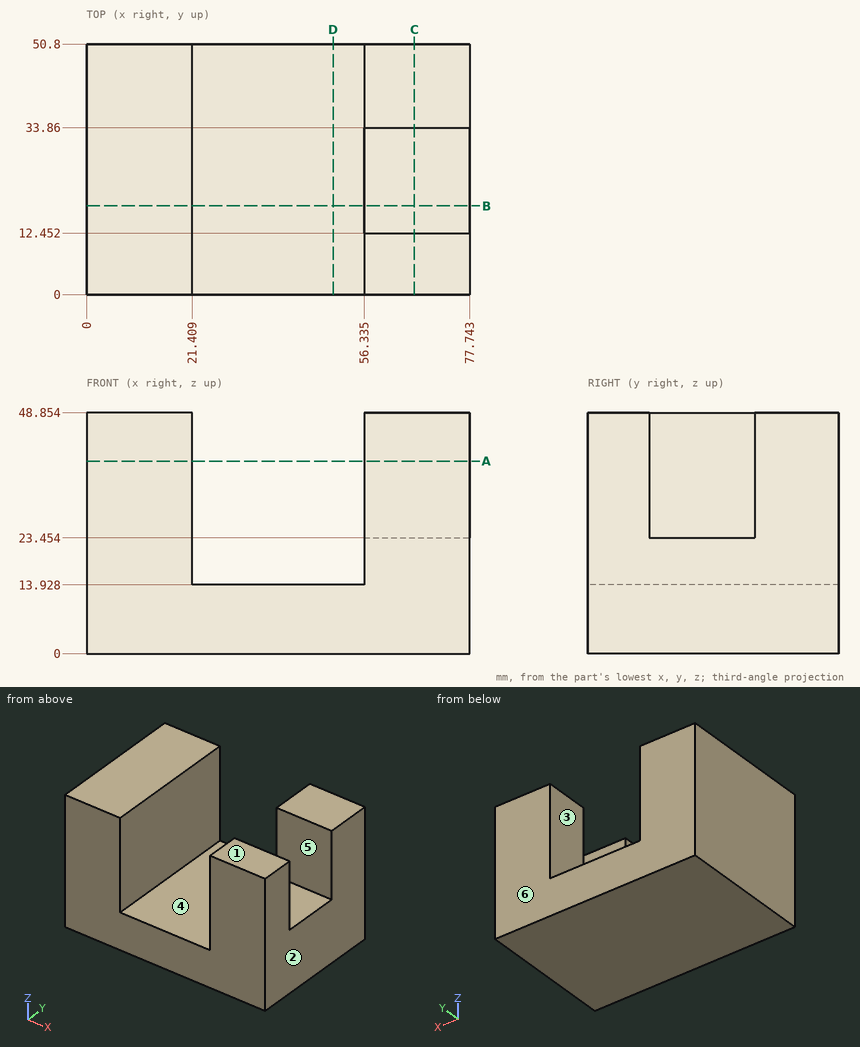
Answer from the drawing. Dimensions are ordinates in mm from the lowest x, y and z of the part. A direction names the side the tool comes from. Round coordinates to 2 decimals unless told otherwise and drop trailing zeros. Order: outer loops, then holes, each group sorted by start corner. A loop starts at its lowest first (then second) coordinate and runs counter-clockwise, first axis right, second up. Notation, with made-up numbers: (30.25, 10.25) -> (70.25, 10.25) arc R20 cw to (70.25, 27.25) -> close; hole circle Ø11 at (0.5, 79.25). An arc over 180 degrees is marked (long way). Answer as CSV lines item,"result".
Q1. Which of the six approach directions +Z, -Z, +X, -X, +Y, -Y give full straight-line access (tool end or side, diameter ignored) to the marked faces 4, 5 and 6?
Computed values:
face 4,"+Z, +Y, -Y"
face 5,"+Z, +X"
face 6,"+Z, -Z, +X, -X, +Y"
Q2. Given pin 1 (10.5 mm diameter, centred on x = 71.5, y = 27, fed in from +Z); pin 2 (6 mm diameter, centred on y = 15.5, z = 41, fed in from +X); pin 3 (1.5 mm diameter, centred on x = 32, y = 17, fed in from +Z), each flat-ended and moving along its own axis, determine where each tip first touches the part or whether it passes through.
Computed values:
pin 1,"stops at z = 23.45"
pin 2,"stops at x = 21.41"
pin 3,"stops at z = 13.93"
Q3. A cutting plane is placed at A-A on z = 39. Determine the outline of the cut face in (x, y) (1 decimal), plus the area to 3 significant figures.
Computed values:
outline,"(0, 0) -> (21.4, 0) -> (21.4, 50.8) -> (0, 50.8) -> close; (56.3, 0) -> (77.7, 0) -> (77.7, 12.5) -> (56.3, 12.5) -> close; (56.3, 33.9) -> (77.7, 33.9) -> (77.7, 50.8) -> (56.3, 50.8) -> close"
area,"1,720 mm^2"
Q4. For a pull along X with two mould halves and no side action, classify the marked faces 1, 2 and 3 as +X half, -X half, draft (parallel to the pull), parting line (faces both ways), or undercut.
Computed values:
face 1,"draft"
face 2,"+X half"
face 3,"undercut"
Q5. Consider line 1 (Y direction, x = 69, z = 42); line 2 (X direction, y = 5.5, z = 23) (1 decimal); line 3 (X direction, y = 30, z = 26). Determine where each line is inside the solid, lowest interval first. Write a range as from..to.
Computed values:
line 1,"y = 0..12.45, 33.86..50.8"
line 2,"x = 0..21.4, 56.3..77.7"
line 3,"x = 0..21.41"
Q6. A cutting plane is placed at B-B on y = 18. Determine the outline of the cut face in (x, z) (1 decimal), plus the area to 3 significant figures.
Computed values:
outline,"(0, 0) -> (77.7, 0) -> (77.7, 23.5) -> (56.3, 23.5) -> (56.3, 13.9) -> (21.4, 13.9) -> (21.4, 48.9) -> (0, 48.9) -> close"
area,"2,030 mm^2"
Q7. A cutting plane is placed at D-D on x = 50. Determine the outline of the cut face in (y, z).
Computed values:
outline,"(0, 0) -> (50.8, 0) -> (50.8, 13.93) -> (0, 13.93) -> close"
Q8. A cutting plane is placed at C-C on x = 66.5. Determine the outline of the cut face in (y, z), plus the area to 3 significant figures.
Computed values:
outline,"(0, 0) -> (50.8, 0) -> (50.8, 48.85) -> (33.86, 48.85) -> (33.86, 23.45) -> (12.45, 23.45) -> (12.45, 48.85) -> (0, 48.85) -> close"
area,"1,940 mm^2"
